Model file for the job. Use its own axes, mm. Face numbers are marked on the shaded views. A direction names the side the tool comes from. Round coordinates to 2 decimals unless told otherwise and drop trailing zeros. Loops run counter-clockwise (first coordinate to the right, second up) from the corner with the lowest first, then second, coordinate; pieces in that order, holes last. Notation, with made-up numbers: M 17.5,-18.5 L 54.5,-18.5 A8 cw 54.5,-4.5 Z; hole C -11,75 d1. An arc over 180 degrees is marked long. Use a Markdown table: item, result. Add a question column.
Q1. Tool access for the marked faces 1 and 2: list every direction of +Z, -Z, +X, -X, +Y, -Y with a clear straight run to the whole face (end or side of a thin tool).
Q2. Cut at D-D (y = -8.5). Give the cut face in (x, z), plus the area to 3 significant figures.
Q3. Pin check, flat tips, straight feed: pin 1 (8 mm diameter, centred on x = -6, y = -1, fed in from -Z); pin 2 (5.5 mm diameter, centred on x = -1, z = 8, fed in from -Y); pin 3 (2 mm diameter, centred on y = -8.5, z = 1.5, fed in from +X); pin 4 (1.5 mm diameter, centred on x = 1, z = 7, fed in from +Y). Stop position of each tip, or through.
Q4. Mould opens along Y. For the marked faces 3, 4 and 5 say: +Y half, -Y half, draft (parallel to the pull), parting line (faces both ways), or undercut.
Q5. Probe line 1 (Y direction, x = 0, z = 2.4); line 2 (Y direction, x = -5, z = 6.25). List the from-to ranges inside material, lowest first. Write a range as from..to.
Q6. Cut at C-C (x = -15). Give the cut face in (y, z).
Q7. Cut at B-B (z = 9.25). Give the cut face in (x, y).
Q8. Cut at A-A (x = 0). Give the cut face in (y, z).
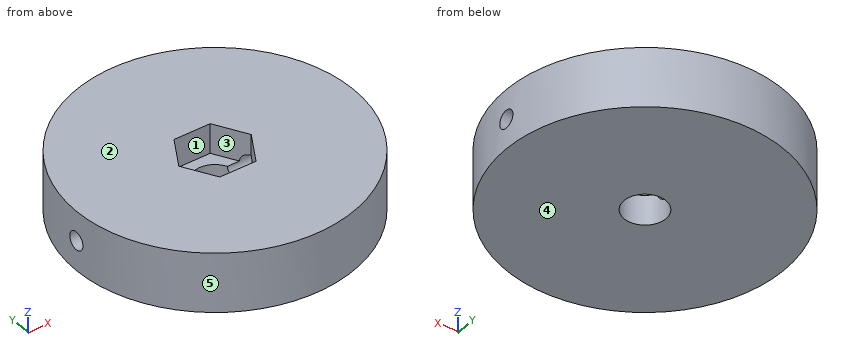
from build123d import *

# Parameters (mm, degrees)
SKETCH_1_R               = 23.25
SKETCH_1_R_2             = 3.5
EXTRUDE_1_DEPTH          = 10
SKETCH_2_R               = 1.5
CUT_EXTRUDE_1_DEPTH      = 24.25
CUT_EXTRUDE_1_DEPTH_BACK = 24.25
CUT_EXTRUDE_3_DEPTH      = 5


with BuildPart() as part:
    # Эскиз1 → Бобышка-Вытянуть1 (new body)
    with BuildSketch(Plane.XY):
        Circle(SKETCH_1_R)
        Circle(SKETCH_1_R_2, mode=Mode.SUBTRACT)
    extrude(amount=EXTRUDE_1_DEPTH)

    # Эскиз2 → Вырез-Вытянуть1 (cut, two sides)
    with BuildSketch(Plane(origin=(0, 0, 0), x_dir=(0, 0, -1), z_dir=(1, 0, 0))) as cut_extrude_1_sk:
        with Locations((-5, 0)):
            Circle(SKETCH_2_R)
    extrude(amount=CUT_EXTRUDE_1_DEPTH, mode=Mode.SUBTRACT)
    extrude(cut_extrude_1_sk.sketch, amount=-CUT_EXTRUDE_1_DEPTH_BACK, mode=Mode.SUBTRACT)

    # Эскиз3 → Вырез-Вытянуть3 (cut)
    with BuildSketch(Plane.XY.offset(10)):
        Polygon((3.031088913, 5.25), (-3.031088913, 5.25), (-6.062177826, 0), (-3.031088913, -5.25), (3.031088913, -5.25), (6.062177826, 0), align=None)
    extrude(amount=-CUT_EXTRUDE_3_DEPTH, mode=Mode.SUBTRACT)


solid = part.part
Checked values:
| question | item | result |
|---|---|---|
| 1 | face 1 | +Z |
| 1 | face 2 | +Z, +X, -X, +Y, -Y |
| 2 | outline | M -21.64,0 L 21.64,0 L 21.64,10 L -21.64,10 Z |
| 2 | area | 433 mm^2 |
| 3 | pin 1 | stops at z = 0 |
| 3 | pin 2 | stops at y = -23.25 |
| 3 | pin 3 | stops at x = 22.01 |
| 3 | pin 4 | stops at y = 23.25 |
| 4 | face 3 | undercut |
| 4 | face 4 | draft |
| 4 | face 5 | parting line |
| 5 | line 1 | y = -23.25..-3.5, 3.5..23.25 |
| 5 | line 2 | y = -22.71..-1.84, 1.84..22.71 |
| 6 | outline | M -17.76,0 L 17.76,0 L 17.76,10 L -17.76,10 Z; hole C 0,5 d3 |
| 7 | outline | C 0,0 d46.5; hole M -6.06,0 L -3.03,-5.25 L 3.03,-5.25 L 6.06,0 L 3.03,5.25 L -3.03,5.25 Z |
| 8 | outline | M -23.25,0 L -3.5,0 L -3.5,5 L -5.25,5 L -5.25,10 L -23.25,10 Z; M 3.5,0 L 23.25,0 L 23.25,10 L 5.25,10 L 5.25,5 L 3.5,5 Z |
